Design review of the part built by this model. Coordinates are the model's own, in mm. A direction names the side the tool comes from. Coordinates: 2 decimals unless noted, no trailing zeros. Order: outer loops, then holes, each group sorted by start corner. A loop starts at its lowest first (then second) coordinate and runs counter-clockwise, first axis right, second up. Notation, with made-up numbers: (47, 20.5) -> (81, 20.5) arc R36 ccw to (81, 57.5) -> close; hole circle Ø10 at (77, 16). An arc over 180 degrees is marked (long way). Write item = value, one per line.
```python
from build123d import *

# Parameters (mm, degrees)
F0_R     = 2.75
F1_DEPTH = 20
F2_SIZE  = 30
F3_R     = 1
F4_R     = 4
F5_SIZE  = 10
F6_W     = 24.290481
F6_H     = 31.840974
F6_W_2   = 17.983475
F6_H_2   = 49.393533
F7_DEPTH = 17
F8_R     = 5


with BuildPart() as f1:
    # F0 (on Front) → F1 (new body)
    with BuildSketch(Plane.XZ):
        with BuildLine():
            ThreePointArc((-5.069714, 17.5), (-14, 3), (-22.930286, 17.5))
            Line((-22.930286, 17.5), (-22.930286, 19))
            Line((-22.930286, 19), (-28, 19))
            Line((-28, 19), (-28, -25))
            Line((-28, -25), (17, -25))
            Line((17, -25), (17, 0))
            Line((17, 0), (0, 0))
            Line((0, 0), (0, 19))
            Line((0, 19), (-5.069714, 19))
            Line((-5.069714, 19), (-5.069714, 17.5))
        make_face()
        with Locations((9, -11.5)):
            Circle(F0_R, mode=Mode.SUBTRACT)
    extrude(amount=F1_DEPTH)

    # F2
    f2_edges = [f1.edges().sort_by_distance(p)[0] for p in [
        (-28, -10, -25),
    ]]
    chamfer(f2_edges, length=F2_SIZE)

    # F3
    f3_edges = [f1.edges().sort_by_distance(p)[0] for p in [
        (0, -10, 0),
    ]]
    fillet(f3_edges, radius=F3_R)

    # F4
    f4_edges = [f1.edges().sort_by_distance(p)[0] for p in [
        (-28, -10, 19),
    ]]
    fillet(f4_edges, radius=F4_R)

    # F5
    f5_edges = [f1.edges().sort_by_distance(p)[0] for p in [
        (9.5, -20, -25),
    ]]
    chamfer(f5_edges, length=F5_SIZE)

    # F6 (on face) → F7 (cut)
    with BuildSketch(Plane.XZ.offset(20)):
        with Locations((-15.14524, -14.920487)):
            Rectangle(F6_W, F6_H)
        with Locations((8.991737, -5.696766)):
            Rectangle(F6_W_2, F6_H_2)
    extrude(amount=-F7_DEPTH, mode=Mode.SUBTRACT)

    # F8
    f8_edges = [f1.edges().sort_by_distance(p)[0] for p in [
        (-3, -11.5, 1),
    ]]
    fillet(f8_edges, radius=F8_R)


solid = f1.part
```
(1) We need section B-B (x = 9). Write out the cut boundary in (y, z), and give its area (3 significant figures).
Report:
outline = (-3, -25) -> (0, -25) -> (0, -14.25) -> (-3, -14.25) -> close; (-3, -8.75) -> (0, -8.75) -> (0, 0) -> (-3, 0) -> close
area = 58.5 mm²
(2) For L1, parallel to X at y = -6.25, z = 13; L2, parallel to Z at x = 9, y = -1.4; L3, parallel to Y at x = 6, z = -21, list the stretches that pass through material, from the lowest coordinate up.
Report:
L1 = -28 to -24, -4 to 0
L2 = -25 to -14.25, -8.75 to 0
L3 = -3 to 0
(3) We need section A-A (z = 13). Write out the cut boundary in (x, y).
Report:
outline = (-28, -20) -> (-24, -20) -> (-24, 0) -> (-28, 0) -> close; (-4, -20) -> (0, -20) -> (0, 0) -> (-4, 0) -> close
(4) We need section D-D (z = -21.5). Write out the cut boundary in (x, y), and give its area (4 significant figures).
Report:
outline = (-1.5, -13.5) -> (0, -13.5) -> (0, -3) -> (17, -3) -> (17, 0) -> (-1.5, 0) -> close
area = 71.25 mm²
(5) For faces 1 (the flat face through (5, -3, -12)), 2 (the flat face through (-16, -12, 1)), 3 (the flat face through (-22.93, -10, 18)), list the 3-axis set-ups (+Z, -Z, +X, -X, +Y, -Y) from which the entire face can be reached by the end or side of a thin tool; tool diameter is ignored.
Report:
face_1 = +Z, -Z, +X, -Y
face_2 = -Z, -X, -Y
face_3 = +Z, +Y, -Y
(6) The part is to be moulded in two halves that separate along Z. For faces 4 (the flat face through (9, -1, 0)), 5 (the flat face through (-28, -10, 10)), 6 (the cylindrical face through (-14, -10, 3)), say which applies: released by +Z, released by -Z, zero draft, split by the parting line, or undercut.
Report:
face_4 = released by +Z
face_5 = zero draft
face_6 = undercut
(7) We need section C-C (y = -18). Write out the cut boundary in (x, z).
Report:
outline = (-28, 5) -> (-24, 1) -> (-8, 1) arc R5 cw to (-3, -4) -> (-3, -17) -> (0, -17) -> (0, 19) -> (-5.07, 19) -> (-5.07, 17.5) arc R10 cw (long way) to (-22.93, 17.5) -> (-22.93, 19) -> (-24, 19) arc R4 ccw to (-28, 15) -> close
(8) Insertion check: pin 1 (5 mm diameter, centred on y = -14.5, z = -14.5, fed in from -X); pin 2 (4 mm diameter, centred on y = -17.5, z = -19.5, fed in from +X); pin 3 (8 mm diameter, centred on x = -1, z = 6, fed in from +Y); pin 4 (6.5 mm diameter, centred on x = -13.5, z = -12.5, fed in from -Y). Each pin has a flat end and moves straight along its axis. Give the tip position at first contact, or say it passes through.
Report:
pin_1 = -3
pin_2 = 0
pin_3 = 0
pin_4 = -3
